Check sheet for the modelled part. Datum: model origin and axes. Units: mm. A direction names the side the tool comes from. Give positions to 0.01 mm unless a question says otherwise; leave off trailing zeros. Order: outer loops, then holes, each group sorted by start corner. A loop starts at its lowest first (then second) coordinate and runs counter-clockwise, first axis right, second up.
Item 1: Gauge pin test, flat ends, axial feed: P1, Ø6, axis at x = 35, z = -10, coming from the +Y side; P2, Ø2, axis at x = 36, z = -12, coming from the -Y side. Record the tip position at first contact, or that the pin passes through.
Item 2: Sectioned sample at A-A on z = -10. Count the separate pieces of the cut face and the enclosed holes in it, and give its area (3 significant figures).
Item 3: Sectioned sample at D-D on y = 4.2. Record the boundary of the cut face in (x, z), and give its area (3 significant figures).
Item 4: Sectioned sample at B-B on x = 21.5. Record the boundary of the cut face in (y, z).
Item 5: Access from +Z, -Z, +X, -X, +Y, -Y to the whole of each face (thin tool, end or side, straight path). Record for faces 1 (the cylindrical face through (20.055, 2.958, -5.321)), 2 (the flat face through (33, 3, -8)).
Item 6: Material ranges on line 1 along X through (y, z) = (5.1, -10); line 2 along X through (y, z) = (1.05, -10); line 3 along Y through (x, z) = (39, -9.5), recorded low to high.
Item 7: Release check for a two-part mould opening along X. For faces 3 (the cylindrical face through (35.78, 4.48, -7.52)), 4 (the flat face through (21, 3, 0)), 5 (the cylindrical face through (42.1, 0.86, -10.14)), 6 (the cylindrical face through (20.055, 2.958, -15.321)) record: released by +X, released by -X, zero draft, split by the parting line, or undercut.
Item 8: Sectioned sample at C-C on x = 8. Record the boundary of the cut face in (y, z).
from build123d import *

# Parameters (mm, degrees)
SKETCH_1_W      = 43
SKETCH_1_H      = 20
SKETCH_1_R      = 5
SKETCH_1_R_2    = 1.48
EXTRUDE_1_DEPTH = 6
EXTRUDE_START   = -3
SKETCH_2_R      = 5
SKETCH_2_R_2    = 2.6
EXTRUDE_2_DEPTH = 3
FILLET_1_R      = 3


with BuildPart() as part:
    # 草图1 → 凸台-拉伸1 (new body)
    with BuildSketch(Plane(origin=(0, 0, 0), x_dir=(1, 0, 0), z_dir=(0, 1, 0))):
        with Locations((21.5, 10)):
            Rectangle(SKETCH_1_W, SKETCH_1_H)
        with Locations(Location((8, 10, 0), (0, 0, 270))):
            Circle(SKETCH_1_R, mode=Mode.SUBTRACT)
        with Locations(Location((35, 10, 0), (0, 0, 270))):
            Circle(SKETCH_1_R, mode=Mode.SUBTRACT)
        with Locations(Location((21.5, 15, 0), (0, 0, 270))):
            Circle(SKETCH_1_R_2, mode=Mode.SUBTRACT)
        with Locations(Location((21.5, 5, 0), (0, 0, 270))):
            Circle(SKETCH_1_R_2, mode=Mode.SUBTRACT)
    extrude(amount=EXTRUDE_1_DEPTH)

    # 草图2 → 凸台-拉伸2 (add)
    # profile 1 of 2: a face of its own
    with BuildSketch(Plane(origin=(0, 6, 0), x_dir=(1, 0, 0), z_dir=(0, 1, 0)).offset(EXTRUDE_START)):
        with Locations(Location((8, 10, 0), (0, 0, 270))):
            Circle(SKETCH_2_R)
        with Locations(Location((8, 10, 0), (0, 0, 270))):
            Circle(SKETCH_2_R_2, mode=Mode.SUBTRACT)
    # profile 2 of 2: a face of its own
    with BuildSketch(Plane(origin=(0, 6, 0), x_dir=(1, 0, 0), z_dir=(0, 1, 0)).offset(EXTRUDE_START)):
        with Locations(Location((35, 10, 0), (0, 0, 270))):
            Circle(SKETCH_2_R)
        with Locations(Location((35, 10, 0), (0, 0, 270))):
            Circle(SKETCH_2_R_2, mode=Mode.SUBTRACT)
    extrude(amount=EXTRUDE_2_DEPTH)

    # 圆角1
    fillet_1_edges = [part.edges().sort_by_distance(p)[0] for p in [
        (43, 0, -10),
        (0, 0, -10),
    ]]
    fillet(fillet_1_edges, radius=FILLET_1_R - 0.0001)  # a hair under: the kernel refuses the full size


solid = part.part
Report:
1. P1: stops at y = 6
1. P2: stops at y = 3
2. separate pieces: 3
2. enclosed holes: 0
2. area: 163 mm2
3. outline: (0, -20) - (43, -20) - (43, 0) - (0, 0) - close; hole circle Ø5.2 at (8, -10); hole circle Ø2.96 at (21.5, -15); hole circle Ø2.96 at (21.5, -5); hole circle Ø5.2 at (35, -10)
3. area: 804 mm2
4. outline: (0, -20) - (6, -20) - (6, -16.48) - (0, -16.48) - close; (0, -13.52) - (6, -13.52) - (6, -6.48) - (0, -6.48) - close; (0, -3.52) - (6, -3.52) - (6, 0) - (0, 0) - close
5. face 1: +Y, -Y
5. face 2: -Y
6. line 1: x = 0 to 5.4, 10.6 to 32.4, 37.6 to 43
6. line 2: x = 0.72 to 3, 13 to 30, 40 to 42.28
6. line 3: y = 3 to 6
7. face 3: undercut
7. face 4: zero draft
7. face 5: released by +X
7. face 6: undercut
8. outline: (0, -20) - (6, -20) - (6, -12.6) - (3, -12.6) - (3, -15) - (0, -15) - close; (0, -5) - (3, -5) - (3, -7.4) - (6, -7.4) - (6, 0) - (0, 0) - close
